Design review of the part shown in the three views and the two pictorial views. Dimensions are in mm from the part's minimum x, y and z. A direction names the side the tool comes from. Coordinates: 2 decimals unless noted, no trailing zeros. Loops run counter-clockwise (first coordinate to the right, second up) from the corner with the lowest first, then second, coordinate; pieces in that order, holes last. Notation, with made-up numbers: (66, 17) -> (119, 17) arc R18 ccw to (119, 38) -> close; hole circle Ø8 at (49, -21). An arc over 180 degrees is marked (long way). One line per item, written item: value. Start each with the question number.
1. Add section D-D on y = 22.5. Write out the cut boundary in (x, z), plus the area to 3 significant figures.
2. Draft analysis for pull direction Y (two halves, no side actions). For the marked faces 1, 2 and 3, state which applies: pulls with the +Y half, pulls with the -Y half, needs draft (parallel to the pull), parting line crosses it, or undercut.
3. For probe 1 along Z at (x, y) = (38, 96); probe 2 along X at (y, z) = (86, 19); probe 3 along Y at (x, z) = (136.5, 44), list the stretches that pass through material, from the lowest coordinate up.
4. Add section C-C on z = 50.8. Write out the cut boundary in (x, y).
5. Insertion check: pin 1 (1 mm diameter, centred on y = 61, z = 51, fed in from +X); pin 2 (6 mm diameter, centred on x = 71, y = 71, fed in from +Z) (3 decimals); pin 3 (10 mm diameter, centred on x = 109.5, y = 20.5, fed in from +Z). Each pin has a flat end and moves straight along its axis. Give the tip position at first contact, or say it passes through.
6. Add section A-A on x = 165.1. Write out the cut boundary in (y, z).
7. Add section B-B on x = 101.6. Write out the cut boundary in (y, z).
8. Machinability: for the marked faces 4 and 5, which of the approach directions +Z, -Z, +X, -X, +Y, -Y give a long, thin tool a straight path to every point of the face, cutting with its end or side? Answer none if there is none.
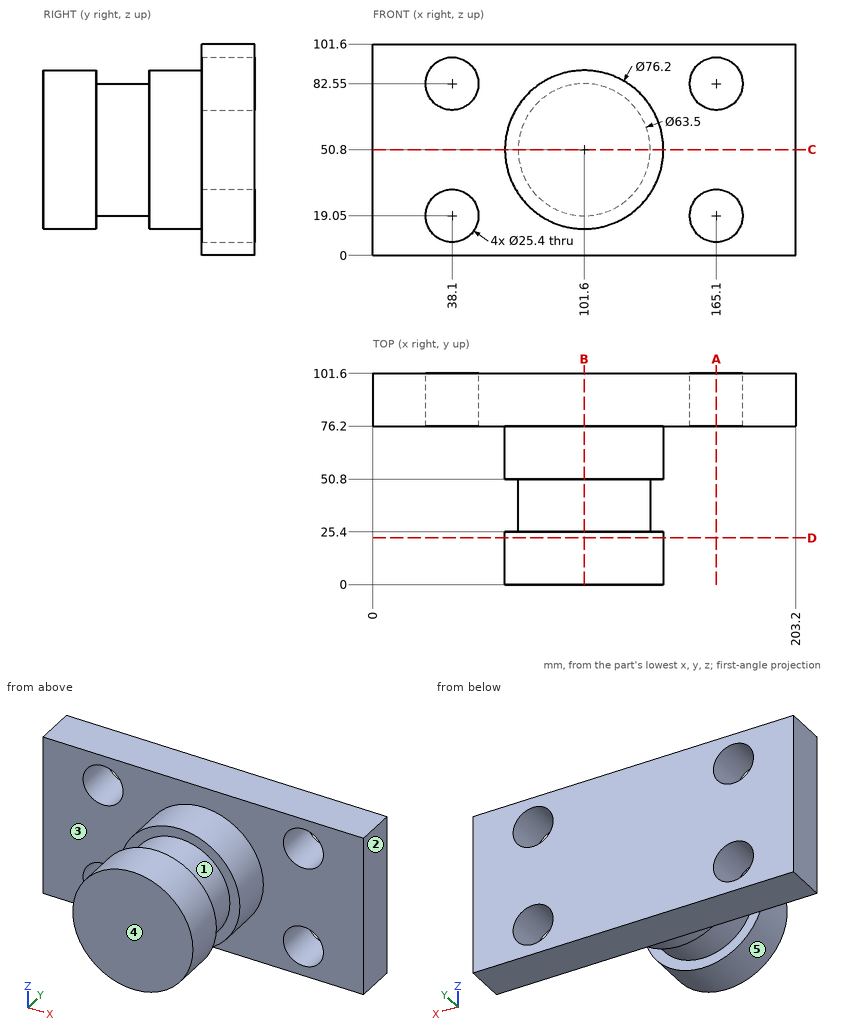
Worked answers:
1. outline: circle Ø76.2 at (101.6, 50.8)
1. area: 4,560 mm²
2. face 1: undercut
2. face 2: needs draft
2. face 3: pulls with the -Y half
3. probe 1: z = 0 to 6.35, 31.75 to 69.85, 95.25 to 101.6
3. probe 2: x = 0 to 25.4, 50.8 to 152.4, 177.8 to 203.2
3. probe 3: y = 0 to 25.4, 50.8 to 101.6
4. outline: (0, 76.2) -> (63.5, 76.2) -> (63.5, 50.8) -> (69.85, 50.8) -> (69.85, 25.4) -> (63.5, 25.4) -> (63.5, 0) -> (139.7, 0) -> (139.7, 25.4) -> (133.35, 25.4) -> (133.35, 50.8) -> (139.7, 50.8) -> (139.7, 76.2) -> (203.2, 76.2) -> (203.2, 101.6) -> (0, 101.6) -> close
5. pin 1: stops at x = 139.7
5. pin 2: stops at z = 77.065
5. pin 3: stops at z = 88.79
6. outline: (76.2, 0) -> (101.6, 0) -> (101.6, 6.35) -> (76.2, 6.35) -> close; (76.2, 31.75) -> (101.6, 31.75) -> (101.6, 69.85) -> (76.2, 69.85) -> close; (76.2, 95.25) -> (101.6, 95.25) -> (101.6, 101.6) -> (76.2, 101.6) -> close
7. outline: (0, 12.7) -> (25.4, 12.7) -> (25.4, 19.05) -> (50.8, 19.05) -> (50.8, 12.7) -> (76.2, 12.7) -> (76.2, 0) -> (101.6, 0) -> (101.6, 101.6) -> (76.2, 101.6) -> (76.2, 88.9) -> (50.8, 88.9) -> (50.8, 82.55) -> (25.4, 82.55) -> (25.4, 88.9) -> (0, 88.9) -> close
8. face 4: +Z, -Z, +X, -X, -Y
8. face 5: -Y
